Could you check a few things on this drawing? It's one solid part, dimensions in mm from its lowest x, y, z. A direction names the side the tool comes from. Give positions to 0.01 mm unless a question says otherwise; leave off trailing zeros. Loops run counter-clockwise (first coordinate to the right, second up) from the corner with the lowest first, then second, coordinate; pieces in that order, holes last. Notation, with made-up numbers: M -5,-30.5 L 18,-30.5 A26 cw 18,4.5 Z; hole C 71,61 d5. An arc over 180 degrees is marked long. Return JSON: item names as keys, results as strings. Group by question number.
1. If we section it at B-B (x = 4.25): Write out the boundary of the cut face in (y, z).
2. For pin 1 (3 mm diameter, centred on x = 3.5, y = 5, fed in from -Z); pin 2 (3 mm diameter, centred on x = 1.5, z = 2.5, fed in from +Y); pin 3 (1.8 mm diameter, centred on x = 2.5, y = 5, fed in from +Z), each with a flat end and sliding along its axis, tell me the tip position at first contact or that it passes through.
3. Please list where these lines run through material, in increasing order: line 1 (Z direction, x = 8.5, y = 1.25); line 2 (Z direction, x = 8.5, y = 3.25); line 3 (Z direction, x = 7.5, y = 5.25).
4. For the marked faces 1, 2, 3, 4 and 5, which set-ups out of +Z, -Z, +X, -X, +Y, -Y let a thin tool reach every point of the face, with its end or its side?
5. If we mould it in two halves opening along Z, with no side actions, what happens to the marked faces 6, 7 and 8? For each: +Z half, -Z half, draft (parallel to the pull), parting line (faces both ways), or undercut.
6. If we section it at D-D (z = 21.25): Write out the boundary of the cut face in (x, y).
7. If we section it at A-A (y = 2.5): Write out the boundary of the cut face in (x, z).
8. If we section it at C-C (y = 4.5): Write out the boundary of the cut face in (x, z).
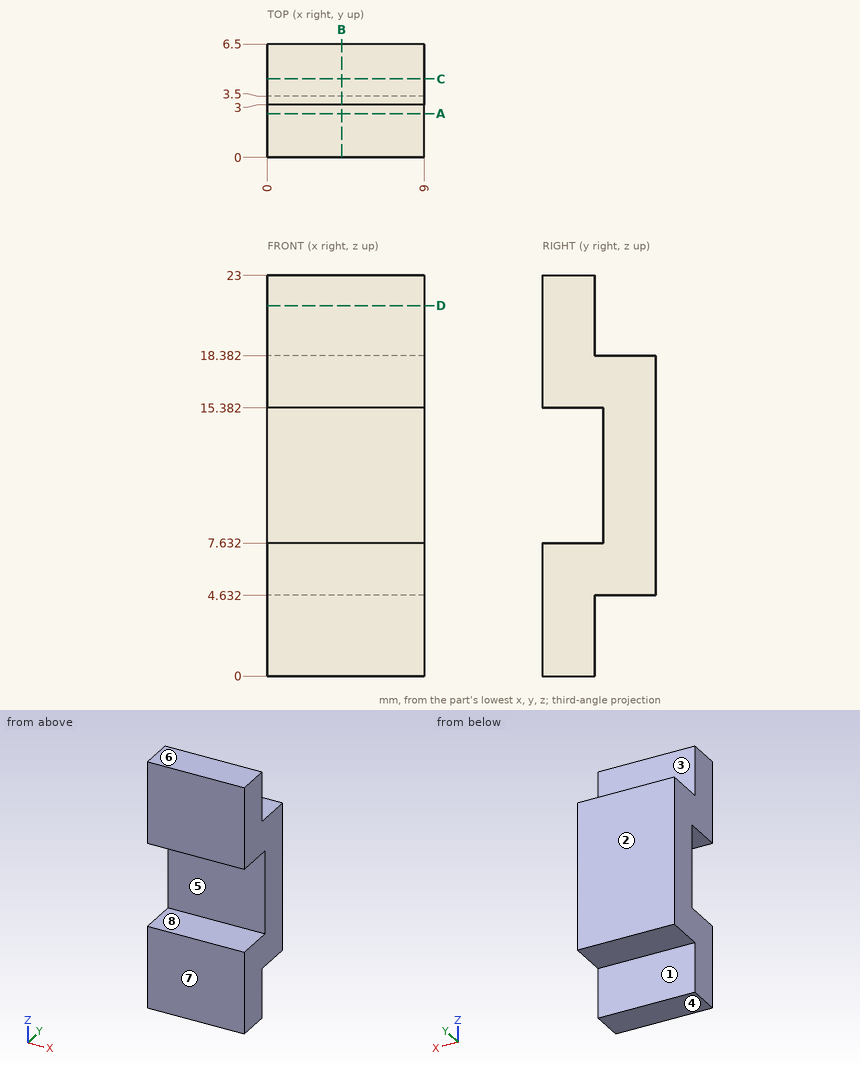
Answer:
{
 "1": {"outline": "M 0,0 L 3,0 L 3,4.63 L 6.5,4.63 L 6.5,18.38 L 3,18.38 L 3,23 L 0,23 L 0,15.38 L 3.5,15.38 L 3.5,7.63 L 0,7.63 Z"},
 "2": {"pin 1": "stops at z = 4.63", "pin 2": "stops at y = 3", "pin 3": "stops at z = 18.38"},
 "3": {"line 1": "z = 0 to 7.63, 15.38 to 23", "line 2": "z = 4.63 to 7.63, 15.38 to 18.38", "line 3": "z = 4.63 to 18.38"},
 "4": {"face 1": "-Z, +X, -X, +Y", "face 2": "+Z, -Z, +X, -X, +Y", "face 3": "+Z, +X, -X, +Y", "face 4": "-Z, +X, -X, +Y, -Y", "face 5": "+X, -X, -Y"},
 "5": {"face 6": "+Z half", "face 7": "draft", "face 8": "undercut"},
 "6": {"outline": "M 0,0 L 9,0 L 9,3 L 0,3 Z"},
 "7": {"outline": "M 0,0 L 9,0 L 9,7.63 L 0,7.63 Z; M 0,15.38 L 9,15.38 L 9,23 L 0,23 Z"},
 "8": {"outline": "M 0,4.63 L 9,4.63 L 9,18.38 L 0,18.38 Z"}
}
